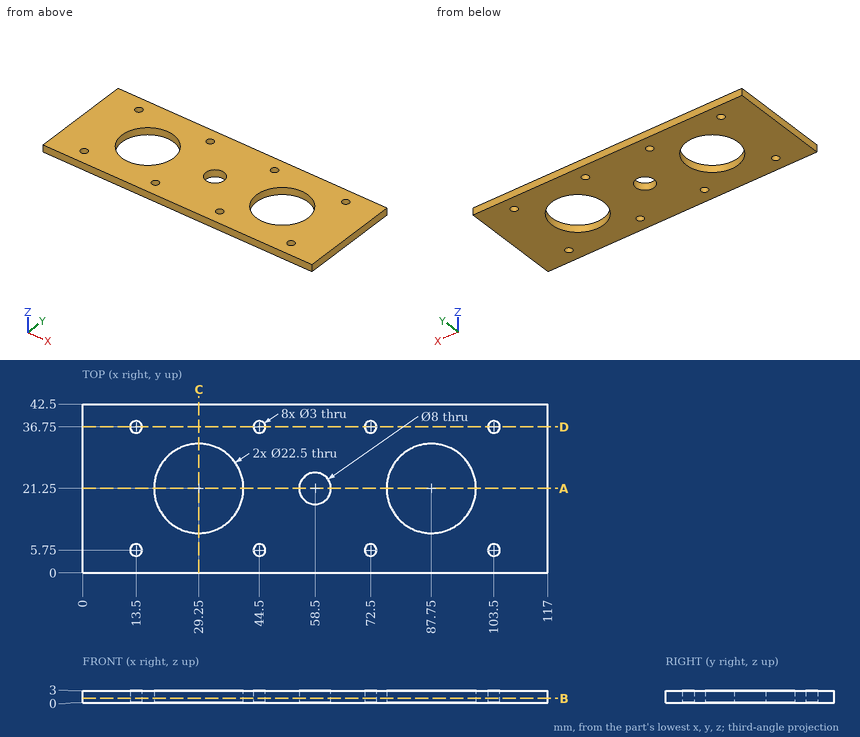
Job drawing, mm, ordinate dimensions from the low corner. One solid piece. Coordinates: 2 decimals unless noted, no trailing zeros. Order: outer loops, then holes, each group sorted by start corner. A loop starts at its lowest first (then second) coordinate and runs counter-clockwise, first axis right, second up. Notation, with made-up numbers: (65.25, 28.5) -> (91.25, 28.5) arc R24 cw to (91.25, 56.5) -> close; hole circle Ø4 at (77.5, -14). An arc over 180 degrees is marked (long way). Return JSON: item names as keys, results as strings. Group by question number.
Item 1: Saw through at B-B on z = 1.15. State how many separate pieces and enclosed holes the cut face has, then the cut area to 3 significant figures.
Item 2: Saw through at D-D on y = 36.75. Write the cut outline in (x, z), then the cut area to 3 significant figures.
Item 3: Saw through at A-A on y = 21.25. Write the cut outline in (x, z), then the cut area to 3 significant figures.
Item 4: Saw through at C-C on x = 29.25. Write the cut outline in (y, z).
Item 5: Wall check: line 1 along Y through (x, z) = (103.5, 1.4); line 2 along X through (y, z) = (37, 0.85); line 3 along X through (y, z) = (11, 0.55). Give the ranges that are in metal, low to high. Write a range as [from, to].
Values found:
{
 "1": {"separate pieces": "1", "enclosed holes": "11", "area": "4,070 mm2"},
 "2": {"outline": "(0, 0) -> (12, 0) -> (12, 3) -> (0, 3) -> close; (15, 0) -> (43, 0) -> (43, 3) -> (15, 3) -> close; (46, 0) -> (71, 0) -> (71, 3) -> (46, 3) -> close; (74, 0) -> (102, 0) -> (102, 3) -> (74, 3) -> close; (105, 0) -> (117, 0) -> (117, 3) -> (105, 3) -> close", "area": "315 mm2"},
 "3": {"outline": "(0, 0) -> (18, 0) -> (18, 3) -> (0, 3) -> close; (40.5, 0) -> (54.5, 0) -> (54.5, 3) -> (40.5, 3) -> close; (62.5, 0) -> (76.5, 0) -> (76.5, 3) -> (62.5, 3) -> close; (99, 0) -> (117, 0) -> (117, 3) -> (99, 3) -> close", "area": "192 mm2"},
 "4": {"outline": "(0, 0) -> (10, 0) -> (10, 3) -> (0, 3) -> close; (32.5, 0) -> (42.5, 0) -> (42.5, 3) -> (32.5, 3) -> close"},
 "5": {"line 1": "y = [0, 4.25], [7.25, 35.25], [38.25, 42.5]", "line 2": "x = [0, 12.02], [14.98, 43.02], [45.98, 71.02], [73.98, 102.02], [104.98, 117]", "line 3": "x = [0, 24.61], [33.89, 83.11], [92.39, 117]"}
}
